Here's the drawing with two shaded views (mm, measured from the low corner). I have some questions. A direction names the side the tool comes from. Coordinates: 2 decimals unless noted, no trailing zeros. Write each loop counter-clockwise with the first axis right and the second up, starting at its lowest first coordinate (ties: lowest second). Pieces come first, ordered by that corner, then holes. Notation, with made-up numbers: (68.5, -1.75) - (96.5, -1.75) arc R24 ccw to (96.5, 8.25) - close; hole circle Ø11 at (-17, -4). An arc over 180 degrees is marked (long way). Answer in a Markdown table with one row per item. Add a question column.
Item 1: Imagine slicing it at B-B (y = 9.5). Please give me the cut outline in (x, z) (1 decimal).
Item 2: Imagine slicing it at A-A (x = 8). Please give me the cut outline in (y, z) (1 decimal).
Item 3: If I drill on probe 1 along Z at (x, y) = (14.5, 4) (1 decimal); probe 2 along Y at (x, z) = (4.5, 7); probe 3 along Z at (x, y) = (1.75, 10.75), over which ranges is the centre line in solid material (lowest first)? Write a range as from..to.
Item 4: I'm going to push flat-ended pins straight in: pin 1 (8 mm diameter, centred on x = 4, y = 4.5, fed in from -Z); pin 2 (8 mm diameter, centred on x = 6, y = 14.5, fed in from +Z). Where does each tip first touch, or does it pass through?
Item 5: Imagine slicing it at C-C (z = 15.5). Please give me the cut outline in (x, y).
Item 6: Which directions (+Z, -Z, +X, -X, +Y, -Y) give clear straight access to the entire face, cutting with the end or side of a thin tool? Please do the marked faces 1, 2 and 3.
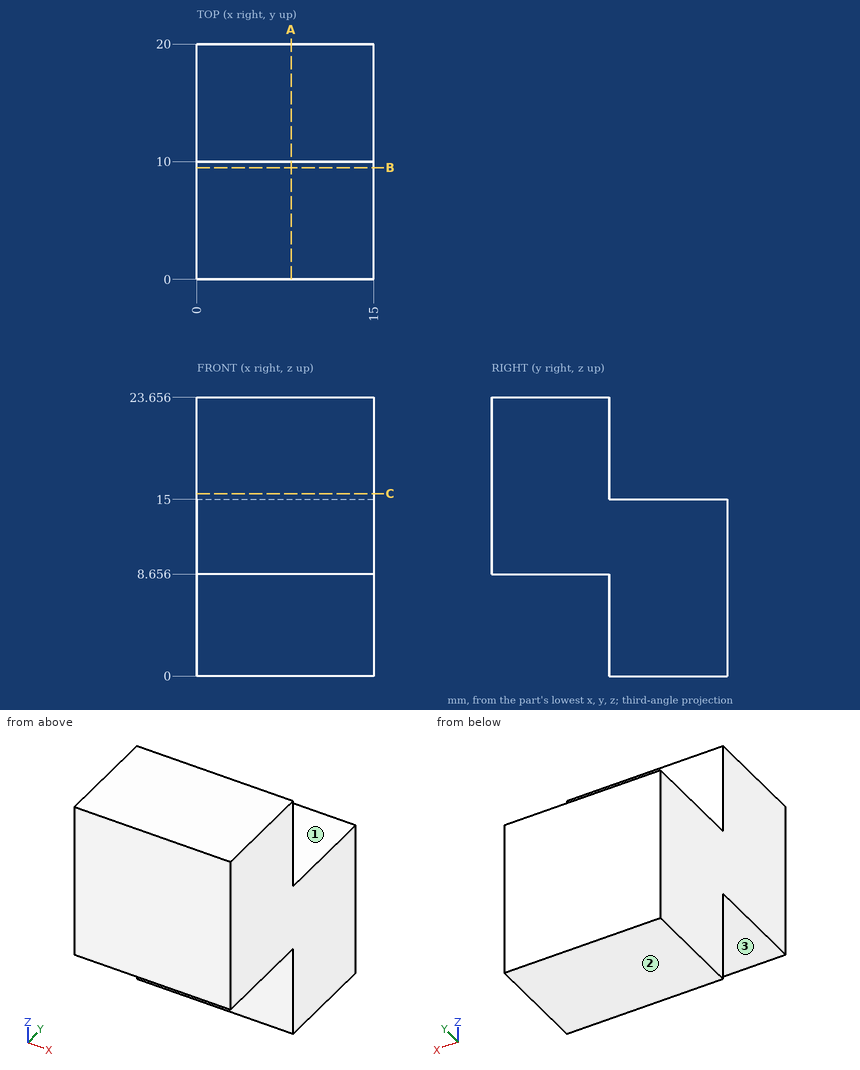
Here are the results:
| question | item | result |
|---|---|---|
| 1 | outline | (0, 8.7) - (15, 8.7) - (15, 23.7) - (0, 23.7) - close |
| 2 | outline | (0, 8.7) - (10, 8.7) - (10, 0) - (20, 0) - (20, 15) - (10, 15) - (10, 23.7) - (0, 23.7) - close |
| 3 | probe 1 | z = 8.7..23.7 |
| 3 | probe 2 | y = 10..20 |
| 3 | probe 3 | z = 0..15 |
| 4 | pin 1 | stops at z = 8.66 |
| 4 | pin 2 | stops at z = 15 |
| 5 | outline | (0, 0) - (15, 0) - (15, 10) - (0, 10) - close |
| 6 | face 1 | +Z, +X, -X, +Y |
| 6 | face 2 | -Z, +X, -X, +Y, -Y |
| 6 | face 3 | -Z, +X, -X, -Y |
